Source: CAD feature listing. Evaluate the final solid. Frame: model axes, mm. Face numbers are marked on the shaded views. A direction names the side the tool comes from. Give positions to 0.01 mm unless a question says otherwise; leave off trailing zeros. Loops run counter-clockwise (first coordinate to the right, second up) from the corner with the lowest first, then second, coordinate; pieces in that order, holes last. Notation, with made-up numbers: M 36.5,15 L 44.5,15 A20 cw 44.5,28 Z; hole C 71.5,3.5 d3. An arc over 180 degrees is marked long. Answer in a Markdown table with one row per item.
```python
from build123d import *

# Parameters (mm, degrees)
F1_DEPTH = 50.8
F0_R     = 4.064
F0_R_2   = 2.54
F2_DEPTH = 19.05
F3_DEPTH = 6.35
F4_DEPTH = 6.35
F5_DEPTH = 6.35


with BuildPart() as f1:
    # F0 (on Top) → F1 (new body)
    with BuildSketch(Plane.XY):
        Polygon((-25.4, -71.196024), (0, -71.196024), (25.4, -71.196024), (25.4, 336.854976), (-25.4, 336.854976), align=None)
        with BuildLine():
            ThreePointArc((3.81, -62.988114), (-2.694077, -65.682191), (0, -59.178114))
            ThreePointArc((0, -59.178114), (2.694077, -60.294037), (3.81, -62.988114))
        make_face(mode=Mode.SUBTRACT)
        Polygon((7.677816, -45.796024), (0.061908, -45.796024), (0.005436, -45.796024), (-7.562184, -45.796024), (-7.562184, -20.396024), (-11.372184, -20.396024), (-11.372184, -1.346024), (-7.562184, -1.346024), (-7.562184, 13.893976), (0.029683, 13.893976), (7.677816, 13.893976), (7.677816, -28.063114), (14.027816, -28.063114), (14.027816, -39.493114), (7.677816, -39.493114), align=None, mode=Mode.SUBTRACT)
        with BuildLine():
            Line((3.871908, 83.696873), (0.058039, 83.696873))
            Line((0.058039, 83.696873), (-3.748092, 83.696873))
            Line((-3.748092, 83.696873), (-3.748092, 97.031873))
            ThreePointArc((-3.748092, 97.031873), (0.061908, 100.841873), (3.871908, 97.031873))
            Line((3.871908, 97.031873), (3.871908, 83.696873))
        make_face(mode=Mode.SUBTRACT)
        Polygon((10.3505, 122.478976), (0, 122.478976), (-10.3505, 122.478976), (-10.3505, 237.159976), (-11.43, 237.159976), (-11.43, 286.054976), (0, 286.054976), (11.43, 286.054976), (11.43, 237.159976), (10.3505, 237.159976), align=None, mode=Mode.SUBTRACT)
    extrude(amount=F1_DEPTH)

    # F0 (on Top) → F2 (join)
    with BuildSketch(Plane.XY):
        Polygon((-11.43, 237.159976), (-10.3505, 237.159976), (10.3505, 237.159976), (11.43, 237.159976), (11.43, 286.054976), (0, 286.054976), (-11.43, 286.054976), align=None)
        with Locations((0, 243.509976)):
            Circle(F0_R, mode=Mode.SUBTRACT)
        with Locations((0, 259.511976)):
            Circle(F0_R_2, mode=Mode.SUBTRACT)
    extrude(amount=F2_DEPTH)

    # F0 (on Top) → F3 (join)
    with BuildSketch(Plane.XY):
        Polygon((0.005436, -45.796024), (0.061908, -45.796024), (7.677816, -45.796024), (7.677816, -39.493114), (14.027816, -39.493114), (14.027816, -28.063114), (7.677816, -28.063114), (7.677816, 13.893976), (0.029683, 13.893976), align=None)
    extrude(amount=F3_DEPTH)

    # F0 (on Top) → F4 (join)
    with BuildSketch(Plane.XY):
        Polygon((-7.562184, -45.796024), (0.005436, -45.796024), (0.029683, 13.893976), (-7.562184, 13.893976), (-7.562184, -1.346024), (-11.372184, -1.346024), (-11.372184, -20.396024), (-7.562184, -20.396024), align=None)
    extrude(amount=F4_DEPTH)

    # F0 (on Top) → F5 (join)
    with BuildSketch(Plane.XY):
        Polygon((0.005436, -45.796024), (0.061908, -45.796024), (7.677816, -45.796024), (7.677816, -39.493114), (14.027816, -39.493114), (14.027816, -28.063114), (7.677816, -28.063114), (7.677816, 13.893976), (0.029683, 13.893976), align=None)
    extrude(amount=F5_DEPTH)


solid = f1.part
```
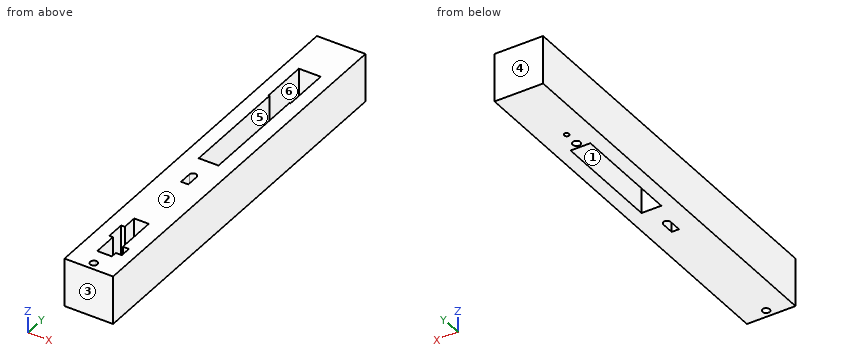
Q1. Contact query for a flat-ended pin moving along its axis: pin 1 Ø7.5 at (x, y) = (-1.5, -27.5) entering from +Z. Output: stop coordinate, or through.
Values follow:
| item | result |
|---|---|
| pin 1 | z = 6.35 |
Q2. Section query C-C (z = 11.5). Output: boundary loops of the cut face in (x, y).
Values follow:
| item | result |
|---|---|
| outline | M -25.4,-71.2 L 25.4,-71.2 L 25.4,336.85 L -25.4,336.85 Z; hole M -11.37,-20.4 L -7.56,-20.4 L -7.56,-45.8 L 7.68,-45.8 L 7.68,-39.49 L 14.03,-39.49 L 14.03,-28.06 L 7.68,-28.06 L 7.68,13.89 L -7.56,13.89 L -7.56,-1.35 L -11.37,-1.35 Z; hole M -10.35,122.48 L 10.35,122.48 L 10.35,237.16 L -10.35,237.16 Z; hole C 0,243.51 d8.13; hole C 0,-62.99 d7.62; hole M -3.75,83.7 L 3.87,83.7 L 3.87,97.03 A3.81 ccw -3.75,97.03 Z; hole C 0,259.51 d5.08 |
Q3. Section query A-A (z = 27). Give the number of separate pieces and of enclosed holes in the cut face, plus the area to 3 significant figures.
Values follow:
| item | result |
|---|---|
| separate pieces | 1 |
| enclosed holes | 4 |
| area | 16,000 mm^2 |
Q4. Ray query, probe 1 along Y at (x, z) = (0, 25); probe 2 along Y at (x, z) = (10, 43.5); probe 3 along X at (y, z) = (170.5, 25). Return the intervals inside material, ascending. Write a range as from..to.
Values follow:
| item | result |
|---|---|
| probe 1 | -71.2..-66.8, -59.18..-45.8, 13.89..83.7, 100.84..122.48, 286.05..336.85 |
| probe 2 | -71.2..-39.49, -28.06..122.48, 286.05..336.85 |
| probe 3 | -25.4..-10.35, 10.35..25.4 |
Q5. Mould query, pull axis Y, two halves, no side actions, for the marked faces 1, 2 and 3. Classes: +Y half, -Y half, draft (parallel to the pull), parting line (faces both ways), or undercut.
Values follow:
| item | result |
|---|---|
| face 1 | undercut |
| face 2 | draft |
| face 3 | -Y half |
Q6. Reachability of the marked faces 4, 5 and 6 from +Z, -Z, +X, -X, +Y, -Y: full face, straight path, thin tool, end or side. Return the list, or none.
Values follow:
| item | result |
|---|---|
| face 4 | +Z, -Z, +X, -X, +Y |
| face 5 | +Z, -Z |
| face 6 | +Z |
Q7. Section query B-B (y = 129.5). Output: boundary loops of the cut face in (x, z).
Values follow:
| item | result |
|---|---|
| outline | M -25.4,0 L -10.35,0 L -10.35,50.8 L -25.4,50.8 Z; M 10.35,0 L 25.4,0 L 25.4,50.8 L 10.35,50.8 Z |
